Can you work these out from the drawing? Everything is in mm from the part's minimum corner. Coordinates: 2 decimals unless noted, no trailing zeros. Loops run counter-clockwise (first coordinate to the right, second up) from the corner with the lowest first, then second, coordinate; pieces in that order, holes last. Notation, with made-up numbers: M 41,-24.75 L 79,-24.75 A17 cw 79,-2.75 Z; hole C 8.5,24 d5. An arc over 180 degrees is marked long. Use CSV: the item, a comma, the result in double quotes. Start each with the question number.
Q1. If we section it at A-A (x = 15): Please give me the cut outline in (y, z).
Q2. If we section it at D-D (y = 15): Please give me the cut outline in (x, z).
Q3. If we section it at C-C (y = 3.5): Please give me the cut outline in (x, z), and give its area (3 significant figures).
Q4. If we section it at B-B (z = 0.8): Please give me the cut outline in (x, y), and give its area (3 significant figures).
Q5. Please list where these lines run through material, in increasing order: probe 1 along Y at (x, z) = (15, 0.45); probe 2 along Y at (x, z) = (14.5, 0.8); probe 3 along X at (y, z) = (6.5, 0.35). Write a range as [from, to].
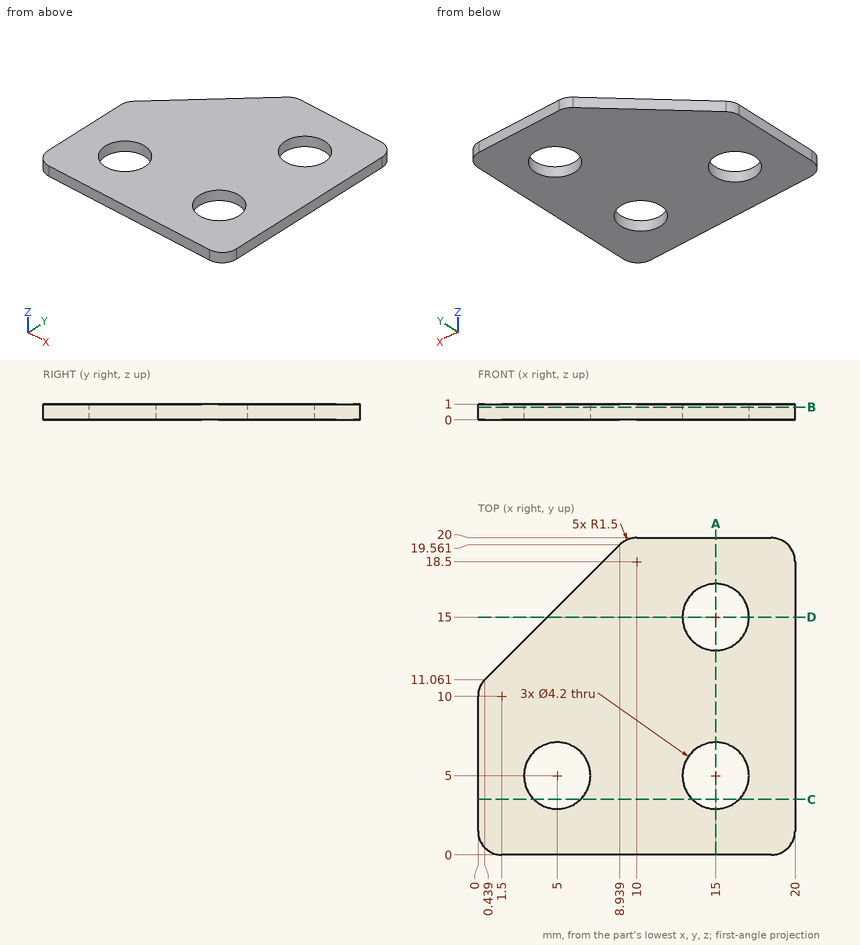
Results below:
1,outline,"M 0,0 L 2.9,0 L 2.9,1 L 0,1 Z; M 7.1,0 L 12.9,0 L 12.9,1 L 7.1,1 Z; M 17.1,0 L 20,0 L 20,1 L 17.1,1 Z"
2,outline,"M 4.38,0 L 12.9,0 L 12.9,1 L 4.38,1 Z; M 17.1,0 L 20,0 L 20,1 L 17.1,1 Z"
3,outline,"M 0,0 L 3.53,0 L 3.53,1 L 0,1 Z; M 6.47,0 L 13.53,0 L 13.53,1 L 6.47,1 Z; M 16.47,0 L 20,0 L 20,1 L 16.47,1 Z"
3,area,"14.1 mm^2"
4,outline,"M 0,1.5 A1.5 ccw 1.5,0 L 18.5,0 A1.5 ccw 20,1.5 L 20,18.5 A1.5 ccw 18.5,20 L 10,20 A1.5 ccw 8.94,19.56 L 0.44,11.06 A1.5 ccw 0,10 Z; hole C 5,5 d4.2; hole C 15,5 d4.2; hole C 15,15 d4.2"
4,area,"313 mm^2"
5,probe 1,"[0, 2.9], [7.1, 12.9], [17.1, 20]"
5,probe 2,"[0, 2.96], [7.04, 12.96], [17.04, 20]"
5,probe 3,"[0, 3.53], [6.47, 13.53], [16.47, 20]"
